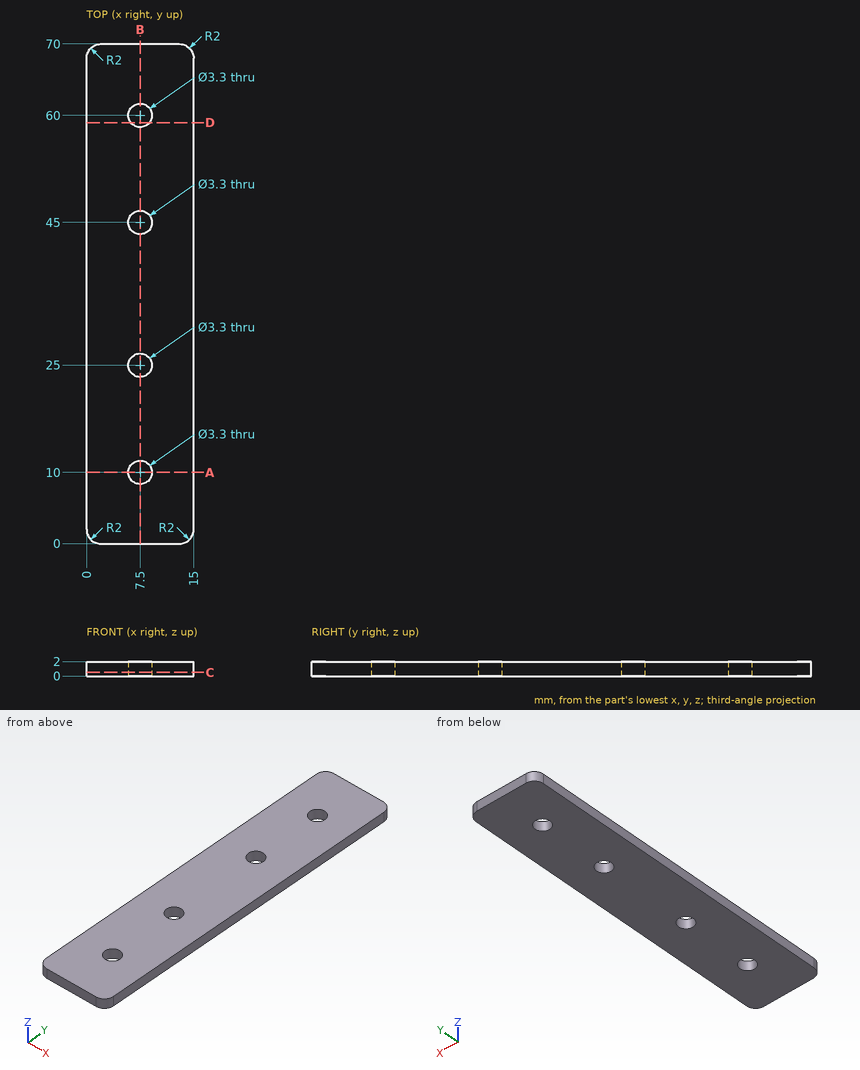
Geometry check sheet. Reference: drawing and pictorial views, mm from the part's lowest x, y, z. Give positions to 0.01 mm unless a question says otherwise; leave off trailing zeros. Order: outer loops, then holes, each group sorted by start corner. A loop starts at its lowest first (then second) coordinate and runs counter-clockwise, first axis right, second up. Notation, with made-up numbers: M 25,-31.5 L 54,-31.5 A23 ccw 54,3.5 Z; hole C -3.5,-8 d10. An arc over 180 degrees is marked long. Answer in a Markdown table with one row per item.
1) Cross-section at D-D, the plane y = 59. Enter the section's corners in (x, z).
Filled sheet:
| item | result |
|---|---|
| outline | M 0,0 L 6.19,0 L 6.19,2 L 0,2 Z; M 8.81,0 L 15,0 L 15,2 L 8.81,2 Z |
2) Cross-section at B-B, the plane x = 7.5. Enter the section's corners in (y, z).
Filled sheet:
| item | result |
|---|---|
| outline | M 0,0 L 8.35,0 L 8.35,2 L 0,2 Z; M 11.65,0 L 23.35,0 L 23.35,2 L 11.65,2 Z; M 26.65,0 L 43.35,0 L 43.35,2 L 26.65,2 Z; M 46.65,0 L 58.35,0 L 58.35,2 L 46.65,2 Z; M 61.65,0 L 70,0 L 70,2 L 61.65,2 Z |
3) Gauge pin test, flat end, axial feed: P1, Ø4.5, axis at x = 7.5, y = 10, coming from the -Z side. Record the tip position at first contact, or that the pin passes through.
Filled sheet:
| item | result |
|---|---|
| P1 | stops at z = 0 |
4) Cross-section at C-C, the plane z = 0.5. Enter the section's corners in (x, y), plus the area to 3 significant figures.
Filled sheet:
| item | result |
|---|---|
| outline | M 0,2 A2 ccw 2,0 L 13,0 A2 ccw 15,2 L 15,68 A2 ccw 13,70 L 2,70 A2 ccw 0,68 Z; hole C 7.5,10 d3.3; hole C 7.5,25 d3.3; hole C 7.5,45 d3.3; hole C 7.5,60 d3.3 |
| area | 1,010 mm2 |
5) Cross-section at A-A, the plane y = 10. Enter the section's corners in (x, z).
Filled sheet:
| item | result |
|---|---|
| outline | M 0,0 L 5.85,0 L 5.85,2 L 0,2 Z; M 9.15,0 L 15,0 L 15,2 L 9.15,2 Z |
6) Thickness scan on L1, parallel to Y at x = 7.5, z = 0.75; L2, parallel to Y at x = 8.5, z = 1.3; L3, parallel to X at y = 9.5, z = 1.65. Record the ranges inside material, lowest first. Write a range as [from, to].
Filled sheet:
| item | result |
|---|---|
| L1 | y = [0, 8.35], [11.65, 23.35], [26.65, 43.35], [46.65, 58.35], [61.65, 70] |
| L2 | y = [0, 8.69], [11.31, 23.69], [26.31, 43.69], [46.31, 58.69], [61.31, 70] |
| L3 | x = [0, 5.93], [9.07, 15] |
